Autodesk Inventor part; units mm, degrees
ref_plane "YZ Plane" through (0, 0, 0) normal (1, 0, 0) x (0, 1, 0)
ref_plane "XZ Plane" through (0, 0, 0) normal (0, 1, 0) x (-1, 0, 0)
ref_plane "XY Plane" through (0, 0, 0) normal (0, 0, 1) x (1, 0, 0)
ref_plane "Work Plane1" through (0, 0, 0) normal (0, 0, 1) x (1, 0, 0)
sketch "Sketch1" plane through (0, 0, 0) normal (0, 0, 1) x (1, 0, 0)
  circle A0 centre (55.8916, -14.7421) radius 1.397 construction
  circle A1 centre (83.8916, 18.2579) radius 1.397 construction
  circle A2 centre (83.8916, -14.7421) radius 1.397 construction
  circle A3 centre (55.8916, 18.2579) radius 1.397 construction
  circle A4 centre (-68.9014, -27.1927) radius 1.905 construction
  circle A5 centre (69.9706, -24.3098) radius 1.905 construction
  arc A6 (-6.1836, 105.2542) -> (-60.0665, 55.7083) centre (-0.9442, 45.4834) ccw construction
  arc A7 (-60.0665, 55.7083) -> (-61.034, 47.7681) centre (-60.6164, 51.7463) ccw construction
  line L0 (-61.034, 47.7681) -> (-68.4839, -23.2145) construction
  arc A8 (-68.4839, -23.2145) -> (-69.2051, -31.1811) centre (-68.9014, -27.1927) ccw construction
  arc A9 (-69.2051, -31.1811) -> (-1.8309, -104.453) centre (0.7162, -34.4994) ccw construction
  arc A10 (-1.8309, -104.453) -> (6.1641, -104.2871) centre (2.169, -104.4843) ccw construction
  arc A11 (6.1641, -104.2871) -> (70.4395, -28.2823) centre (0.7162, -34.4994) ccw construction
  arc A12 (70.4395, -28.2823) -> (69.3883, -20.3524) centre (69.9706, -24.3098) ccw construction
  line L1 (69.3883, -20.3524) -> (69.0778, -18.2421) construction
  line L2 (87.8916, -18.2421) -> (69.0778, -18.2421) construction
  line L3 (87.8916, 21.7579) -> (87.8916, -18.2421) construction
  line L4 (63.1925, 21.7579) -> (87.8916, 21.7579) construction
  line L5 (63.1925, 21.7579) -> (58.999, 50.2599) construction
  arc A13 (58.999, 50.2599) -> (57.7029, 58.1531) centre (58.4167, 54.2173) ccw construction
  arc A14 (57.7029, 58.1531) -> (1.8102, 105.4201) centre (-0.9442, 45.4834) ccw construction
  arc A15 (1.8102, 105.4201) -> (-6.1836, 105.2542) centre (-2.1895, 105.4705) ccw construction
  circle A16 centre (58.4167, 54.2173) radius 1.905 construction
  circle A17 centre (-2.1895, 105.4705) radius 1.905 construction
  circle A18 centre (-60.6164, 51.7463) radius 1.905 construction
  circle A19 centre (2.169, -104.4843) radius 1.905 construction
  circle A20 centre (-0.9442, 45.4834) radius 6.75 construction
  circle A21 centre (75.8916, -7.1378) radius 4
  circle A22 centre (66.7556, 10.6536) radius 4
  line L6 (87.8916, -18.2421) -> (87.8916, 21.7579)
  line L7 (87.8916, 21.7579) -> (49.8916, 21.7579)
  line L8 (49.8916, 21.7579) -> (49.8916, -18.2421)
  line L9 (49.8916, -18.2421) -> (87.8916, -18.2421)
  circle A23 centre (83.8916, -14.7421) radius 1.905
  circle A24 centre (55.8916, -14.7421) radius 1.905
  circle A25 centre (55.8916, 18.2579) radius 1.905
  circle A26 centre (83.8916, 18.2579) radius 1.905
  point P0 (0, 0)
  dimension "d0" = 3.81
  dimension "d1" = 38
extrude "Extrusion1" add sketch "Sketch1" along normal blind 5
sketch "Sketch2" plane through (0, 0, 5) normal (0, 0, 1) x (1, 0, 0)
  circle A0 centre (66.7556, 10.6536) radius 4 construction
  circle A1 centre (75.8916, -7.1378) radius 4 construction
  circle A2 centre (83.8916, 18.2579) radius 1.905 construction
  circle A3 centre (55.8916, 18.2579) radius 1.905 construction
  circle A4 centre (55.8916, -14.7421) radius 1.905 construction
  circle A5 centre (83.8916, -14.7421) radius 1.905 construction
  line L0 (87.8916, -18.2421) -> (87.8916, 21.7579) construction
  line L1 (87.8916, 21.7579) -> (49.8916, 21.7579) construction
  line L2 (49.8916, 21.7579) -> (49.8916, -18.2421) construction
  line L3 (49.8916, -18.2421) -> (87.8916, -18.2421) construction
  line L4 (87.8916, -18.2421) -> (49.8916, -18.2421)
  line L5 (49.8916, -18.2421) -> (49.8916, -16.6471)
  line L6 (49.8916, -16.6471) -> (87.8916, -16.6471)
  line L7 (87.8916, -16.6471) -> (87.8916, -18.2421)
  line L8 (87.8916, 21.7579) -> (49.8916, 21.7579)
  line L9 (87.8916, 21.7579) -> (49.8916, 21.7579)
  line L10 (49.8916, 21.7579) -> (49.8916, 20.1629)
  line L11 (49.8916, 20.1629) -> (87.8916, 20.1629)
  line L12 (87.8916, 20.1629) -> (87.8916, 21.7579)
  line L13 (49.8916, -16.6471) -> (53.9866, -16.6471)
  line L14 (53.9866, -16.6471) -> (53.9866, 20.1629)
  line L15 (53.9866, 20.1629) -> (49.8916, 20.1629)
  line L16 (49.8916, 20.1629) -> (49.8916, -16.6471)
  circle A6 centre (55.8916, -14.7421) radius 1.905
  point P0 (0, 0)
extrude "Extrusion2" add sketch "Sketch2" along normal blind 50 contours L4 L5 L6 L7 | L16 L11 L14 L6 | L10 L8 L12 L11
sketch "Sketch3" plane through (0, 0, 55) normal (0, 0, 1) x (1, 0, 0)
  line L0 (55.8916, -16.6471) -> (83.8916, -16.6471)
  circle A0 centre (83.8916, -14.7421) radius 1.905
  line L1 (83.8916, -16.6471) -> (87.8916, -16.6471)
  line L2 (87.8916, -16.6471) -> (87.8916, 20.1629)
  line L3 (87.8916, 20.1629) -> (83.8916, 20.1629)
  circle A1 centre (83.8916, 18.2579) radius 1.905
  line L4 (83.8916, 20.1629) -> (55.8916, 20.1629)
  arc A2 (53.9866, 18.2579) -> (55.8916, 20.1629) centre (55.8916, 18.2579) ccw
  line L5 (53.9866, 18.2579) -> (53.9866, -14.7421)
  arc A3 (55.8916, -16.6471) -> (53.9866, -14.7421) centre (55.8916, -14.7421) ccw
  circle A4 centre (66.7556, 10.6536) radius 4
  circle A5 centre (75.8916, -7.1378) radius 4
  line L6 (53.9866, 20.1629) -> (87.8916, 20.1629)
  line L7 (87.8916, 20.1629) -> (87.8916, 21.7579)
  line L8 (87.8916, 21.7579) -> (49.8916, 21.7579)
  line L9 (49.8916, 21.7579) -> (49.8916, -18.2421)
  line L10 (49.8916, -18.2421) -> (87.8916, -18.2421)
  line L11 (87.8916, -18.2421) -> (87.8916, -16.6471)
  line L12 (87.8916, -16.6471) -> (53.9866, -16.6471)
  line L13 (53.9866, -16.6471) -> (53.9866, 20.1629)
  point P0 (0, 0)
extrude "Extrusion3" add sketch "Sketch3" along normal blind 5 contours A3 L5 A2 L4 L3 L2 L1 L0 | L0 L1 L11 L10 L9 L8 L7 L3 L4 L6 L13 L5 L12
sketch "Sketch4" plane through (87.8916, -18.2421, 0) normal (1, 0, 0) x (0, 0, -1)
  line L0 (-5, 38.405) -> (-55, 38.405)
  line L1 (-5, 1.595) -> (-5, 38.405)
  line L2 (-5, 1.595) -> (-55, 1.595)
  line L3 (-55, 1.595) -> (-55, 38.405)
  line L4 (0, 40) -> (-60, 40)
  line L5 (-60, 0) -> (-60, 40)
  line L6 (0, 0) -> (-60, 0)
  line L7 (0, 0) -> (0, 40)
  point P0 (0, 18.2421)
extrude "Extrusion4" add sketch "Sketch4" along normal blind 5
sketch "Sketch5" plane through (0, 0, 5) normal (0, 0, 1) x (1, 0, 0)
  line L0 (55.8916, -16.6471) -> (83.8916, -16.6471)
  circle A0 centre (83.8916, -14.7421) radius 1.905
  line L1 (83.8916, -16.6471) -> (92.8916, -16.6471)
  line L2 (92.8916, 20.1629) -> (92.8916, -16.6471)
  line L3 (92.8916, 20.1629) -> (83.8916, 20.1629)
  circle A1 centre (83.8916, 18.2579) radius 1.905
  line L4 (83.8916, 20.1629) -> (55.8916, 20.1629)
  arc A2 (53.9866, 18.2579) -> (55.8916, 20.1629) centre (55.8916, 18.2579) ccw
  line L5 (53.9866, 18.2579) -> (53.9866, -14.7421)
  arc A3 (55.8916, -16.6471) -> (53.9866, -14.7421) centre (55.8916, -14.7421) ccw
  circle A4 centre (66.7556, 10.6536) radius 4
  circle A5 centre (75.8916, -7.1378) radius 4
  line L6 (59.9866, 20.1629) -> (59.9866, 13.1536)
  line L7 (59.9866, 13.1536) -> (53.9866, 13.1536)
  line L8 (53.9866, 8.1536) -> (59.9866, 8.1536)
  line L9 (59.9866, 8.1536) -> (59.9866, -4.6378)
  line L10 (59.9866, -4.6378) -> (53.9866, -4.6378)
  line L11 (53.9866, -9.6378) -> (59.9866, -9.6378)
  line L12 (59.9866, -9.6378) -> (59.9866, -16.6471)
  line L13 (59.9866, -9.6378) -> (59.9866, -4.6378) construction
  line L14 (59.9866, 8.1536) -> (59.9866, 13.1536) construction
  point P0 (0, 0)
  point P1 (59.9866, -7.1378)
  point P2 (59.9866, 10.6536)
  dimension "d10" = 5
  dimension "d11" = 6
  dimension "d12" = 5
extrude "Extrusion5" add sketch "Sketch5" along normal up to next contours A3 L5 L11 L12 L0 | L5 L8 L9 L10 | L5 A2 L4 L6 L7
sketch "Sketch6" plane through (92.8916, -18.2421, 0) normal (1, 0, 0) x (0, 0, -1)
  line L0 (-5, 38.405) -> (-5, 1.595) construction
  line L1 (-5, 1.595) -> (-55, 1.595) construction
  line L2 (-55, 1.595) -> (-55, 38.405) construction
  line L3 (-55, 38.405) -> (-5, 38.405) construction
  line L4 (0, 40) -> (-60, 40) construction
  line L5 (-60, 40) -> (-60, 0) construction
  line L6 (-60, 0) -> (0, 0) construction
  line L7 (0, 0) -> (0, 40) construction
  line L8 (-60, 0) -> (0, 0) construction
  line L9 (-30, 0) -> (-30, 40) construction
  line L10 (-52.5, 45) -> (-7.5, 45) construction
  line L11 (-7.5, 45) -> (-7.5, -5) construction
  line L12 (-7.5, -5) -> (-52.5, -5) construction
  line L13 (-52.5, -5) -> (-52.5, 45) construction
  line L14 (-52.5, 45) -> (-7.5, -5) construction
  line L15 (-7.5, 45) -> (-52.5, -5) construction
  circle A0 centre (-7.5, -5) radius 1.397
  circle A1 centre (-52.5, -5) radius 1.397
  circle A2 centre (-7.5, 45) radius 1.397
  circle A3 centre (-52.5, 45) radius 1.397
  line L16 (-7.5, -5) -> (-7.5, 0) construction
  line L17 (-11.5, -5) -> (-11.5, 0)
  line L18 (-3.5, 0) -> (-3.5, -5)
  arc A4 (-11.5, -5) -> (-3.5, -5) centre (-7.5, -5) ccw
  arc A5 (-3.5, 0) -> (-11.5, 0) centre (-7.5, 0) ccw construction
  line L19 (-52.5, -5) -> (-52.5, 0) construction
  line L20 (-48.5, -5) -> (-48.5, 0)
  line L21 (-56.5, 0) -> (-56.5, -5)
  arc A6 (-56.5, -5) -> (-48.5, -5) centre (-52.5, -5) ccw
  arc A7 (-48.5, 0) -> (-56.5, 0) centre (-52.5, 0) ccw construction
  line L22 (-52.5, 45) -> (-52.5, 40) construction
  line L23 (-48.5, 45) -> (-48.5, 40)
  line L24 (-56.5, 40) -> (-56.5, 45)
  arc A8 (-48.5, 45) -> (-56.5, 45) centre (-52.5, 45) ccw
  arc A9 (-56.5, 40) -> (-48.5, 40) centre (-52.5, 40) ccw construction
  line L25 (-7.5, 45) -> (-7.5, 40) construction
  line L26 (-11.5, 45) -> (-11.5, 40)
  line L27 (-3.5, 40) -> (-3.5, 45)
  arc A10 (-3.5, 45) -> (-11.5, 45) centre (-7.5, 45) ccw
  arc A11 (-11.5, 40) -> (-3.5, 40) centre (-7.5, 40) ccw construction
  line L28 (-3.5, 0) -> (-11.5, 0)
  line L29 (-56.5, 0) -> (-48.5, 0)
  line L30 (-56.5, 40) -> (-48.5, 40)
  line L31 (0, 40) -> (-60, 40)
  line L32 (-11.5, 40) -> (-3.5, 40)
  point P0 (0, 18.2421)
  point P1 (-30, 20)
  point P2 (-7.5, -2.5)
  point P3 (-52.5, -2.5)
  point P4 (-52.5, 42.5)
  point P5 (-7.5, 42.5)
  dimension "d15" = 2.794
  dimension "d16" = 50
  dimension "d17" = 45
  dimension "d18" = 4
extrude "Extrusion6" add sketch "Sketch6" against normal blind 10
properties part number "shifter box 1"
Geometry check sheet. Reference: the model listing, model coordinates, mm. A direction names the side the tool comes from. Coordinates: 2 decimals unless noted, no trailing zeros. Order: outer loops, then holes, each group sorted by start corner. A loop starts at its lowest first (then second) coordinate and runs counter-clockwise, first axis right, second up. Notation, with made-up numbers: (-0.75, -7) - (48.25, -7) arc R17 ccw to (48.25, 24) - close; hole circle Ø7 at (-8.5, 0.5). An arc over 180 degrees is marked (long way). Answer in a Markdown table with one row per item. Add a question column.
1) Set-up check for faces 3 (the flat face through (73, 2, 55)), 4 (the flat face through (88, -21, 3.5)), 5 (the flat face through (55, 20.163, 32)): record each of +Z, -Z, +X, -X, +Y, -Y from which the full face is reachable in a straight line by a thin tool's end or side.
2) Gauge pin test, flat ends, axial feed: P1, Ø6.5, axis at x = 57, z = 29.5, coming from the +Y side; P2, Ø4, axis at x = 86.5, y = -22, coming from the -Z side; P3, Ø2, axis at y = 19, z = 22.5, coming from the +X side; P4, Ø3.5, axis at x = 55.89, y = 18.26, coming from the -Z side. Record the tip position at first contact, or that the pin passes through.
3) Cross-section at A-A, the plane z = 7.5. State how many separate pieces and enclosed holes the cut face has, then the cut area to 3 significant figures.
4) Material ranges on line 1 along Y through (x, z) = (59, 15); line 2 along Y through (x, z) = (67.5, 47); line 3 along Y through (x, z) = (89, 7.5), recorded low to high. Write a range as [from, to].
5) Release check for a two-part mould opening along Y. For faces 1 (the flat face through (82.892, 25, 8)), 2 (the flat face through (76, -16.647, 30)) record: +Y half, -Y half, draft (parallel to the pull), parting line (faces both ways), or undercut.
6) Cross-section at C-C, the plane x = 65. Record the cut outline in (y, z).
7) Cross-section at B-B, the plane x = 59. Record the cut outline in (y, z), then the cut area to 3 significant figures.
Check result:
| question | item | result |
|---|---|---|
| 1 | face 3 | +X |
| 1 | face 4 | -Z, +X, -X, -Y |
| 1 | face 5 | +Z |
| 2 | P1 | stops at y = 21.76 |
| 2 | P2 | stops at z = 3.5 |
| 2 | P3 | stops at x = 59.99 |
| 2 | P4 | passes through |
| 3 | separate pieces | 3 |
| 3 | enclosed holes | 2 |
| 3 | area | 549 mm² |
| 4 | line 1 | y = [-18.24, -9.64], [-4.64, 8.15], [13.15, 21.76] |
| 4 | line 2 | y = [-18.24, -16.65], [20.16, 21.76] |
| 4 | line 3 | y = [-27.24, -24.64], [-21.85, -16.65], [20.16, 25.36], [28.15, 30.76] |
| 5 | face 1 | draft |
| 5 | face 2 | undercut |
| 6 | outline | (-18.24, 0) - (7.06, 0) - (7.06, 5) - (-16.65, 5) - (-16.65, 55) - (7.06, 55) - (7.06, 60) - (-18.24, 60) - close; (14.25, 0) - (21.76, 0) - (21.76, 60) - (14.25, 60) - (14.25, 55) - (20.16, 55) - (20.16, 5) - (14.25, 5) - close |
| 7 | outline | (-18.24, 0) - (21.76, 0) - (21.76, 60) - (-18.24, 60) - close; hole (-9.64, 5) - (-4.64, 5) - (-4.64, 55) - (-9.64, 55) - close; hole (8.15, 5) - (13.15, 5) - (13.15, 55) - (8.15, 55) - close |
| 7 | area | 1,900 mm² |
